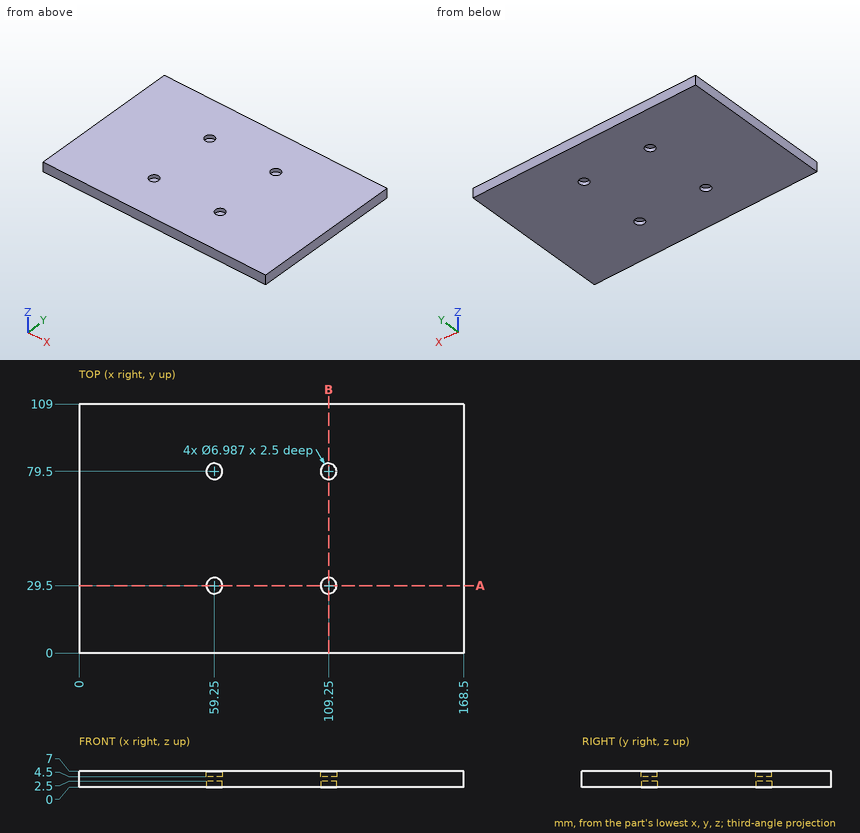
Design review of the part shown in the three views and the two pictorial views. Dimensions are in mm from the part's minimum x, y and z. Round coordinates to 2 decimals unless told otherwise and drop trailing zeros. Loops run counter-clockwise (first coordinate to the right, second up) from the corner with the lowest first, then second, coordinate; pieces in that order, holes last. Notation, with made-up numbers: (37, 7) - (76, 7) arc R27 ccw to (76, 38) - close; hole circle Ø9 at (-12, -3). An arc over 180 degrees is marked (long way). Write each question's results on one line, items separated by ' | '. Start each with the question number.
Q1. Take a section at A-A on y = 29.5. Give the boundary of the cut face in (x, z), plus the area to 3 significant figures.
Q2. Insertion check: P1, Ø4, axis at x = 59.25, y = 29.5, coming from the +Z side; P2, Ø2, axis at x = 109, y = 29.5, coming from the -Z side. Each pin has a flat end and moves straight along its axis. Give the tip position at first contact, or say it passes through.
Q3. Take a section at B-B on x = 109.25. Give the boundary of the cut face in (y, z).
Q4. Wall thickness on line 1 along Y through (x, z) = (59.25, 5.15); line 2 along Z through (x, y) = (111, 78): over which ranges is each line inside the solid? List them lowest first. Write a range as [from, to].
Data:
1) outline: (0, 0) - (55.76, 0) - (55.76, 2.5) - (62.74, 2.5) - (62.74, 0) - (105.76, 0) - (105.76, 2.5) - (112.74, 2.5) - (112.74, 0) - (168.5, 0) - (168.5, 7) - (112.74, 7) - (112.74, 4.5) - (105.76, 4.5) - (105.76, 7) - (62.74, 7) - (62.74, 4.5) - (55.76, 4.5) - (55.76, 7) - (0, 7) - close | area: 1,110 mm²
2) P1: stops at z = 4.5 | P2: stops at z = 2.5
3) outline: (0, 0) - (26.01, 0) - (26.01, 2.5) - (32.99, 2.5) - (32.99, 0) - (76.01, 0) - (76.01, 2.5) - (82.99, 2.5) - (82.99, 0) - (109, 0) - (109, 7) - (82.99, 7) - (82.99, 4.5) - (76.01, 4.5) - (76.01, 7) - (32.99, 7) - (32.99, 4.5) - (26.01, 4.5) - (26.01, 7) - (0, 7) - close
4) line 1: y = [0, 26.01], [32.99, 76.01], [82.99, 109] | line 2: z = [2.5, 4.5]
